Design review of the part built by this model. Coordinates are the model's own, in mm. A direction names the side the tool comes from. Round coordinates to 2 decimals unless told otherwise and drop trailing zeros. Loops run counter-clockwise (first coordinate to the right, second up) from the corner with the lowest first, then second, coordinate; pieces in that order, holes last. Notation, with made-up numbers: M 79,45.5 L 131,45.5 A16 ccw 131,53.5 Z; hole C -17.75,2 d4. An arc over 180 degrees is marked long. Use a Markdown table: item, result.
from build123d import *

# Parameters (mm, degrees)
SKETCH1_W               = 65
SKETCH1_H               = 65
BOSS_EXTRUDE1_DEPTH     = 24
SKETCH3_W               = 21.5
SKETCH3_H               = 22
CUT_EXTRUDE2_DEPTH      = 25
SKETCH4_R               = 2.5
CUT_EXTRUDE3_DEPTH      = 33.5
CUT_EXTRUDE3_DEPTH_BACK = 33.5


with BuildPart() as part:
    # Sketch1 → Boss-Extrude1 (new body)
    with BuildSketch(Plane(origin=(0, 0, 0), x_dir=(1, 0, 0), z_dir=(0, 1, 0))):
        Rectangle(SKETCH1_W, SKETCH1_H)
    extrude(amount=BOSS_EXTRUDE1_DEPTH)

    # Sketch3 → Cut-Extrude2 (cut, through all)
    with BuildSketch(Plane(origin=(0, 24, 0), x_dir=(1, 0, 0), z_dir=(0, 1, 0))):
        with Locations((-21.75, 21.5)):
            Rectangle(SKETCH3_W, SKETCH3_H)
        with Locations((21.75, 21.5)):
            Rectangle(SKETCH3_W, SKETCH3_H)
        with Locations((21.75, -21.5)):
            Rectangle(SKETCH3_W, SKETCH3_H)
        with Locations((-21.75, -21.5)):
            Rectangle(SKETCH3_W, SKETCH3_H)
    extrude(amount=-CUT_EXTRUDE2_DEPTH, mode=Mode.SUBTRACT)

    # Sketch4 → Cut-Extrude3 (cut, two sides)
    with BuildSketch(Plane.XY) as cut_extrude3_sk:
        with Locations((-22.25, 13)):
            Circle(SKETCH4_R)
        with Locations((22.25, 13)):
            Circle(SKETCH4_R)
    extrude(amount=CUT_EXTRUDE3_DEPTH, mode=Mode.SUBTRACT)
    extrude(cut_extrude3_sk.sketch, amount=-CUT_EXTRUDE3_DEPTH_BACK, mode=Mode.SUBTRACT)


solid = part.part
1. Take a section at A-A on x = -22.25. Give the boundary of the cut face in (y, z), and give its area (3 significant figures).
Check values:
| item | result |
|---|---|
| outline | M 0,-10.5 L 10.5,-10.5 L 10.5,10.5 L 0,10.5 Z; M 15.5,-10.5 L 24,-10.5 L 24,10.5 L 15.5,10.5 Z |
| area | 399 mm² |
2. Take a section at C-C on y = 16.5. Give the boundary of the cut face in (x, z).
Check values:
| item | result |
|---|---|
| outline | M -32.5,-10.5 L -11,-10.5 L -11,-32.5 L 11,-32.5 L 11,-10.5 L 32.5,-10.5 L 32.5,10.5 L 11,10.5 L 11,32.5 L -11,32.5 L -11,10.5 L -32.5,10.5 Z |
3. Insertion check: pin 1 (11 mm diameter, centred on x = -17, y = 8, fed in from -Z); pin 2 (4 mm diameter, centred on x = 22.25, y = 13, fed in from +Z); pin 3 (6.5 mm diameter, centred on x = -18, y = 17.5, fed in from +Z); pin 4 (8 mm diameter, centred on x = -11.5, z = 18, fed in from -Y). Each pin has a flat end and moves straight along its axis. Give the tip position at first contact, or say it passes through.
Check values:
| item | result |
|---|---|
| pin 1 | stops at z = -10.5 |
| pin 2 | passes through |
| pin 3 | stops at z = 10.5 |
| pin 4 | stops at y = 0 |
4. Machinability: for faces 1 (the face through (11, 12, -21)), 2 (the face through (-19.5, 12.2, 10.5)), 3 (the face through (-19.5, 12.2, -10.5)), which of the approach directions +Z, -Z, +X, -X, +Y, -Y give a long, thin tool a straight path to every point of the face, cutting with its end or side? Answer none if there is none.
Check values:
| item | result |
|---|---|
| face 1 | -Z, +X, +Y, -Y |
| face 2 | +Z, -X, +Y, -Y |
| face 3 | -Z, -X, +Y, -Y |
5. Wall thickness on line 1 along X through (y, z) = (13, 0.5); line 2 along Y through (x, z) = (22.25, 1); line 3 along Z through (x, y) = (-15.5, 2.75): over which ranges is each line inside the solid? List them lowest first. Write a range as from..to.
Check values:
| item | result |
|---|---|
| line 1 | x = -32.5..-24.75, -19.75..19.75, 24.75..32.5 |
| line 2 | y = 0..10.5, 15.5..24 |
| line 3 | z = -10.5..10.5 |
6. Take a section at D-D on z = -21. Give the boundary of the cut face in (x, y).
Check values:
| item | result |
|---|---|
| outline | M -11,0 L 11,0 L 11,24 L -11,24 Z |
7. The part is to be moulded in two halves that separate along X. For faces 4 (the face through (20.266, 11.479, 0.147)), 5 (the face through (19, 12, 10.5)), 6 (the face through (11, 12, 22)), say which applies: pulls with the +X half, pulls with the -X half, needs draft (parallel to the pull), parting line crosses it, or undercut.
Check values:
| item | result |
|---|---|
| face 4 | undercut |
| face 5 | needs draft |
| face 6 | pulls with the +X half |
8. Take a section at B-B on y = 13. Give the boundary of the cut face in (x, z).
Check values:
| item | result |
|---|---|
| outline | M -32.5,-10.5 L -24.75,-10.5 L -24.75,10.5 L -32.5,10.5 Z; M -19.75,-10.5 L -11,-10.5 L -11,-32.5 L 11,-32.5 L 11,-10.5 L 19.75,-10.5 L 19.75,10.5 L 11,10.5 L 11,32.5 L -11,32.5 L -11,10.5 L -19.75,10.5 Z; M 24.75,-10.5 L 32.5,-10.5 L 32.5,10.5 L 24.75,10.5 Z |
